Model file for the job. Use its own axes, mm. Face numbers are marked on the shaded views. A direction names the side the tool comes from. Give positions to 0.01 mm unless a question says otherwise; leave off trailing zeros. Loops run counter-clockwise (first coordinate to the right, second up) from the corner with the lowest first, then second, coordinate; pieces in that order, holes last. Notation, with made-up numbers: (89, 37) -> (148, 37) arc R12 cw to (148, 59) -> close; hole circle Ø6 at (-12.5, 3). An arc over 180 degrees is marked (long way). Use CSV: the item, a comma, the result in double quotes. Start each with the question number.
(1) Drill centre lines: probe 1 along X at (y, z) = (-7.5, 43.5); probe 2 along Y at (x, z) = (-32, 49.5); probe 3 along Y at (x, z) = (84.5, -18). Where is each one in solid material? Low to high.
(2) Cut at C-C on y = -121.5. Write the cut outline in (x, z).
(3) Cut at A-A on z = 34. Write the cut outline in (x, y).
(4) Pull direction X, two halves, no side cores. Call the marked faces 4, 5 and 6: pulls with the +X half, pulls with the -X half, needs draft (parallel to the pull), parting line crosses it, or undercut.
(5) 3-axis set-ups, long thin cutter, end or side, ignore diameter. For the marked faces 1, 2 and 3: which of +Z, -Z, +X, -X, +Y, -Y reach the whole face in a straight line?
(6) Cut at D-D on z = 12. Write the cut outline in (x, y), then the cut area to 3 significant figures.
(7) Flat gauge pins, fed straight in: pin 1 (3 mm diameter, centred on x = 16.5, y = 6.5, fed in from -Z); pin 2 (16 mm diameter, centred on y = -218.5, z = 36.5, fed in from -X); pin 3 (15.5 mm diameter, centred on y = 68, z = 44.5, fed in from +X). Where does each tip first touch, or does it go through?
(8) Cut at B-B on x = -3.5. Write the cut outline in (y, z).
from build123d import *

# Parameters (mm, degrees)
F0_W     = 320
F0_H     = 370
F1_DEPTH = 70
F2_W     = 282
F2_H     = 332
F3_DEPTH = 51
F4_W     = 342
F4_H     = 140
F4_W_2   = 320
F4_H_2   = 70
F5_DEPTH = 19
F6_W     = 100
F6_H     = 20
F7_DEPTH = 20


with BuildPart() as f1:
    # F0 (on Top) → F1 (new body)
    with BuildSketch(Plane.XY):
        Rectangle(F0_W, F0_H)
    extrude(amount=F1_DEPTH)

    # F2 (on face) → F3 (cut)
    with BuildSketch(Plane.XY.offset(70)):
        Rectangle(F2_W, F2_H)
    extrude(amount=-F3_DEPTH, mode=Mode.SUBTRACT)

    # F4 (on face) → F5 (join)
    with BuildSketch(Plane.XZ.offset(185)):
        with Locations((0, 35)):
            Rectangle(F4_W, F4_H)
        with Locations((0, 35)):
            Rectangle(F4_W_2, F4_H_2, mode=Mode.SUBTRACT)
        with Locations((0, 35)):
            Rectangle(F4_W_2, F4_H_2)
    extrude(amount=F5_DEPTH)

    # F6 (on face) → F7 (join)
    with BuildSketch(Plane.XZ.offset(204)):
        with Locations((0, 35)):
            Rectangle(F6_W, F6_H)
    extrude(amount=F7_DEPTH)


solid = f1.part
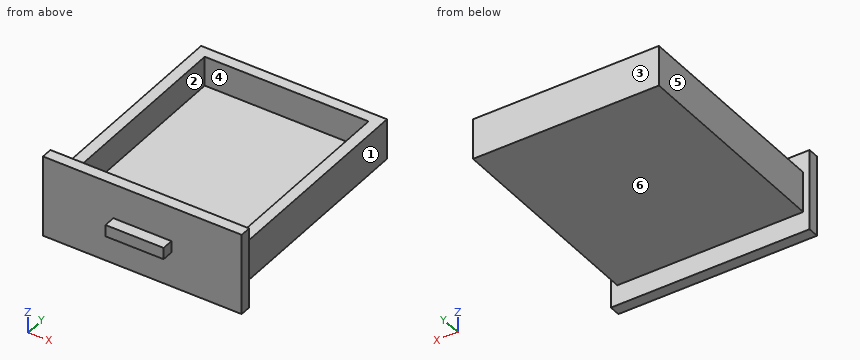
Check result:
1,probe 1,"-160 to -141, 141 to 160"
1,probe 2,"-204 to -166, 166 to 185"
1,probe 3,"-204 to -185"
2,outline,"(-160, 0) -> (160, 0) -> (160, 70) -> (141, 70) -> (141, 19) -> (-141, 19) -> (-141, 70) -> (-160, 70) -> close"
3,outline,"(-171, -204) -> (-50, -204) -> (-50, -224) -> (50, -224) -> (50, -204) -> (171, -204) -> (171, -185) -> (160, -185) -> (160, 185) -> (-160, 185) -> (-160, -185) -> (-171, -185) -> close; hole (-141, -166) -> (141, -166) -> (141, 166) -> (-141, 166) -> close"
4,face 4,"undercut"
4,face 5,"pulls with the -X half"
4,face 6,"needs draft"
5,face 1,"+Z, -Z, +X, +Y"
5,face 2,"+Z"
5,face 3,"+Z, -Z, +X, -X, +Y"
6,outline,"(-171, -204) -> (171, -204) -> (171, -185) -> (160, -185) -> (160, 185) -> (-160, 185) -> (-160, -185) -> (-171, -185) -> close"
6,area,"125,000 mm²"
7,pin 1,"z = 0"
7,pin 2,"x = -50"
7,pin 3,"x = 160"
8,outline,"(-224, 25) -> (-204, 25) -> (-204, -35) -> (-185, -35) -> (-185, 0) -> (185, 0) -> (185, 70) -> (166, 70) -> (166, 19) -> (-166, 19) -> (-166, 70) -> (-185, 70) -> (-185, 105) -> (-204, 105) -> (-204, 45) -> (-224, 45) -> close"
